Autodesk Inventor part; units mm, degrees
ref_plane "YZ Plane" through (0, 0, 0) normal (1, 0, 0) x (0, 1, 0)
ref_plane "XZ Plane" through (0, 0, 0) normal (0, 1, 0) x (-1, 0, 0)
ref_plane "XY Plane" through (0, 0, 0) normal (0, 0, 1) x (1, 0, 0)
sketch "Sketch1" plane through (0, 0, 0) normal (0, 1, 0) x (-1, 0, 0)
  line L0 (-39.2837, 182.0907) -> (45.1561, 182.0907)
  line L1 (45.1561, 182.0907) -> (45.1561, 192.9873)
  line L2 (-39.2837, 192.9873) -> (-39.2837, 182.0907)
  circle A0 centre (40.7951, 187.539) radius 2.2274
  circle A1 centre (-34.9227, 187.539) radius 2.2274
  line L3 (52.1157, -152.8547) -> (52.1157, 254.4851) construction
  line L4 (-39.2837, 182.0907) -> (45.1561, 182.0907) construction
  line L5 (45.1561, 182.0907) -> (45.1561, 192.9873) construction
  line L6 (45.1561, 192.9873) -> (-39.2837, 192.9873)
  line L7 (-39.2837, 192.9873) -> (-39.2837, 182.0907) construction
  circle A2 centre (40.7951, 187.539) radius 2.2274
  circle A3 centre (-34.9227, 187.539) radius 2.2274
  line L8 (-47.9603, 254.4851) -> (-47.9603, -152.8547) construction
  line L9 (45.1561, 166.5182) -> (-39.2837, 166.5182)
  line L10 (-39.2837, 166.5182) -> (-39.2837, 155.6216)
  line L11 (-39.2837, 155.6216) -> (45.1561, 155.6216)
  line L12 (45.1561, 155.6216) -> (45.1561, 166.5182)
  circle A4 centre (40.7951, 161.0699) radius 2.2274
  circle A5 centre (-34.9227, 161.0699) radius 2.2274
  point P0 (0, 0)
  point P1 (0, 0)
  point P2 (0, 0)
  dimension "d0" = 84.4398
  dimension "d1" = 10.8966
  dimension "d3" = 2.1336
  dimension "d4" = 2.1336
  dimension "d5" = 6.9596
  dimension "d6" = 84.4398
  dimension "d7" = 10.8966
  dimension "d9" = 2.1336
  dimension "d10" = 2.1336
  dimension "d14" = 10.8966
  dimension "d15" = 3.2209
  dimension "d16" = 3.2209
  dimension "d17" = 2.1336
  dimension "d18" = 2.1336
  dimension "d19" = 3.2209
  dimension "d20" = 3.2209
  dimension "d21" = 75.7178
  dimension "d22" = 75.7178
  dimension "d23" = 84.4398
extrude "Extrusion1" add sketch "Sketch1" along normal blind 29.0322 contours L12 L11 L10 L9
chamfer "Chamfer1" distance 12.7 angle 45 2 edges at (39.2837, 29.0322, 161.0699) (-45.1561, 29.0322, 161.0699)
equation "\"d4\" = d3"
equation "\"d10\" = d9"
equation "\"d14\" = d7"
equation "\"d17\" = d9"
equation "\"d18\" = d10"
equation "\"d19\" = d15"
equation "\"d20\" = d16"
properties part number "Voltage Divider (Rough)"
CAD build for the part. Positions are in the model's coordinates, mm. Round coordinates to 2 decimals unless told otherwise and drop trailing zeros. Loops run counter-clockwise (first coordinate to the right, second up) from the corner with the lowest first, then second, coordinate; pieces in that order, holes last. Notation, with made-up numbers: (26.5, 51.5) - (69.5, 51.5) arc R11 ccw to (69.5, 55.5) - close; hole circle Ø3 at (71.5, 32.5). An arc over 180 degrees is marked (long way). Return JSON: item names as keys, results as strings. Group by question number.
Q1. Band-saw the part on A-A on y = 20.5. Give the cut face in (x, z), plus the area to 3 significant figures.
Q2. Drill centre lines: line 1 along X through (y, z) = (7.5, 161.25) (3 decimals); line 2 along X through (y, z) = (8.25, 162); line 3 along Z through (x, y) = (-40, 14.75). Where is each one in solid material? Low to high. Write a range as [from, to].
Q3. Flat gauge pins, fed straight in: pin 1 Ø1.5 at (y, z) = (19.5, 163.5) entering from +X; pin 2 Ø3.5 at (x, z) = (34.92, 161.07) entering from -Y. Where does each tip first touch, or does it go through?
Q4. Band-saw the part on D-D on y = 26.75. Give the cut face in (x, z).
Q5. Band-saw the part on B-B on z = 156.5. Give the cut face in (x, y), plus the area to 3 significant figures.
Q6. Two-plate mould, pull along X, no slides. Class faces 1 (the face through (-2, 0, 161)), 2 (the face through (39.284, 8, 161)), 3 (the face through (32.8, 11.3, 160.4)), 4 (the face through (-38.57, 11.31, 160.97)): +X half, -X half, draft (parallel to the pull), parting line (faces both ways), or undercut.
Q7. Band-saw the part on C-C on y = 12.75. Give the cut face in (x, z).
Solutions:
{
 "1": {"outline": "(-40.99, 155.62) - (35.12, 155.62) - (35.12, 158.85) arc R2.23 cw (long way) to (35.12, 163.29) - (35.12, 166.52) - (-40.99, 166.52) - (-40.99, 163.29) arc R2.23 cw (long way) to (-40.99, 158.85) - close", "area": "812 mm^2"},
 "2": {"line 1": "x = [-45.156, -43.015], [-38.575, 32.703], [37.143, 39.284]", "line 2": "x = [-45.16, -42.82], [-38.77, 32.9], [36.95, 39.28]", "line 3": "z = [155.62, 158.99], [163.15, 166.52]"},
 "3": {"pin 1": "stops at x = 36.87", "pin 2": "passes through"},
 "4": {"outline": "(-34.74, 155.62) - (28.87, 155.62) - (28.87, 166.52) - (-34.74, 166.52) - close"},
 "5": {"outline": "(-45.16, 0) - (39.28, 0) - (39.28, 16.33) - (26.58, 29.03) - (-32.46, 29.03) - (-45.16, 16.33) - close", "area": "2,290 mm^2"},
 "6": {"face 1": "draft", "face 2": "+X half", "face 3": "undercut", "face 4": "undercut"},
 "7": {"outline": "(-45.16, 155.62) - (39.28, 155.62) - (39.28, 166.52) - (-45.16, 166.52) - close; hole circle Ø4.45 at (-40.8, 161.07); hole circle Ø4.45 at (34.92, 161.07)"}
}
